Answer from the drawing. Dimensions are ordinates in mm from the lowest x, y and z of the part. A direction names the side the tool comes from. Give positions to 0.01 mm unless a question says otherwise; leave off trailing zeros. Loops run counter-clockwise (first coordinate to the right, second up) from the corner with the lowest first, then second, coordinate; pieces in that order, holes last. Notation, with made-up numbers: M 25.25,31 L 35.25,31 A34 cw 35.25,69 Z; hole C 0.5,22 d8. An arc over 180 degrees is marked long. Use a Markdown table: item, result.
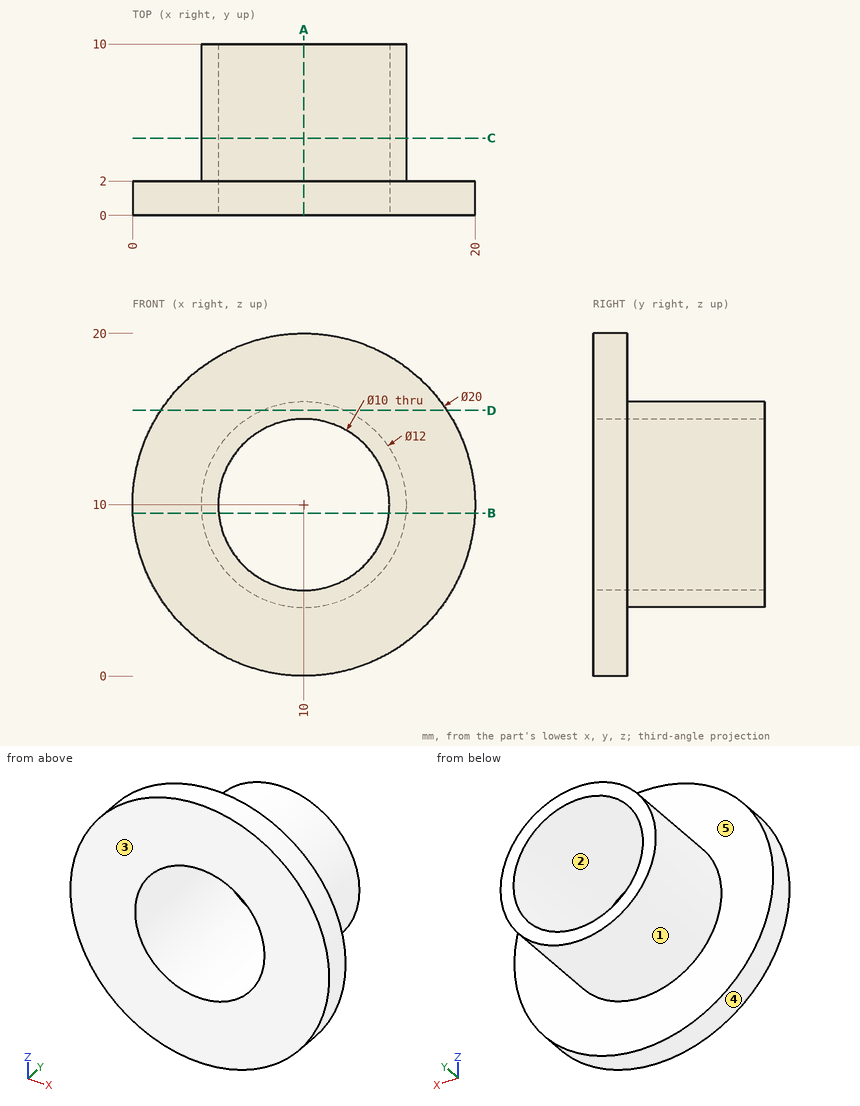
(1) The mould has two halves that part along Z. Classify the marked faces 1, 2 and 3: released by +Z, released by -Z, zero draft, split by the parting line, or undercut.
Entries:
| item | result |
|---|---|
| face 1 | split by the parting line |
| face 2 | undercut |
| face 3 | zero draft |
(2) Which of the six approach directions +Z, -Z, +X, -X, +Y, -Y give full straight-line access (tool end or side, diameter ignored) to the marked faces 4 and 5?
Entries:
| item | result |
|---|---|
| face 4 | +Y, -Y |
| face 5 | +Y |
(3) Consider probe 1 along Z at (x, y) = (10, 4); probe 2 along Z at (x, y) = (12.75, 0.75); probe 3 along Y at (x, z) = (5, 14.25). Determine where each line is inside the solid, lowest interval first. Write a range as [from, to].
Entries:
| item | result |
|---|---|
| probe 1 | z = [4, 5], [15, 16] |
| probe 2 | z = [0.39, 5.82], [14.18, 19.61] |
| probe 3 | y = [0, 2] |
(4) A cutting plane is placed at D-D (z = 15.5). Write down the section's boundary in (x, y), and give its area (3 significant figures).
Entries:
| item | result |
|---|---|
| outline | M 1.65,0 L 18.35,0 L 18.35,2 L 12.4,2 L 12.4,10 L 7.6,10 L 7.6,2 L 1.65,2 Z |
| area | 71.8 mm² |
(5) A cutting plane is placed at C-C (y = 4.5). Write down the section's boundary in (x, z), and give its area (3 significant figures).
Entries:
| item | result |
|---|---|
| outline | C 10,10 d12; hole C 10,10 d10 |
| area | 34.6 mm² |
(6) A cutting plane is placed at B-B (z = 9.5). Write down the section's boundary in (x, y), and give its area (3 significant figures).
Entries:
| item | result |
|---|---|
| outline | M 0.01,0 L 5.03,0 L 5.03,10 L 4.02,10 L 4.02,2 L 0.01,2 Z; M 14.97,0 L 19.99,0 L 19.99,2 L 15.98,2 L 15.98,10 L 14.97,10 Z |
| area | 36.1 mm² |
(7) A cutting plane is placed at A-A (x = 10). Write down the section's boundary in (y, z), and give its area (3 significant figures).
Entries:
| item | result |
|---|---|
| outline | M 0,0 L 2,0 L 2,4 L 10,4 L 10,5 L 0,5 Z; M 0,15 L 10,15 L 10,16 L 2,16 L 2,20 L 0,20 Z |
| area | 36.0 mm² |
(8) Given P1, Ø1, axis at x = 3, z = 7, coming from the +Y side; P2, Ø2, axis at x = 13, z = 7.5, coming from the +Y side; P3, Ø6, axis at x = 8.5, y = 5.5, coming from the -Z side; P4, Ø1, axis at x = 5.5, y = 3, coming from the -Z side, each flat-ended and moving along its own axis, determine where each tip first touches the part or whether it passes through.
Entries:
| item | result |
|---|---|
| P1 | stops at y = 2 |
| P2 | passes through |
| P3 | stops at z = 4 |
| P4 | stops at z = 5.53 |
